Could you check a few things on this drawing? It's one solid part, dimensions in mm from its lowest x, y, z. A direction names the side the tool comes from. Give positions to 0.01 mm unless a question says otherwise; leave off trailing zeros. Loops run counter-clockwise (first coordinate to the right, second up) from the corner with the lowest first, then second, coordinate; pieces in that order, holes last.
Q1. Suppose I cut it at C-C (y = 1.6). List the corners of the cut face in (x, z) for me.
Q2. Suppose I cut it at D-D (x = 18.5). List the corners of the cut face in (y, z) for me.
Q3. Suppose I cut it at B-B (x = 3.5). List the corners of the cut face in (y, z) for me, and give its area (3 significant figures).
Q4. I need wall thicknesses on probe 1 along X at (y, z) = (1.6, 3.5); probe 2 along Z at (x, y) = (22, 1.8); probe 3 along X at (y, z) = (0.9, 6.5). Which ranges of each line are inside material? Lowest first, please.
Q5. Thinking about a two-plate mould opening in X: for the marked faces 1 and 2, which applies, pulls with the +X half, pulls with the -X half, needs draft (parallel to the pull), parting line crosses it, or undercut?
Q6. Suppose I cut it at A-A (z = 3.5). List the corners of the cut face in (x, y) for me, and give its area (3 significant figures).
Q7. I'm going to push flat-ended pins straight in: P1, Ø2, axis at x = 8.5, z = 4, coming from the -Y side; P2, Ø5, axis at x = 26, z = 9, coming from the +Y side. Where does each tip first touch, or does it pass through?
Q8. For the marked faces 3 and 4, which set-ups out of +Z, -Z, +X, -X, +Y, -Y let a thin tool reach every point of the face, with its end or its side?
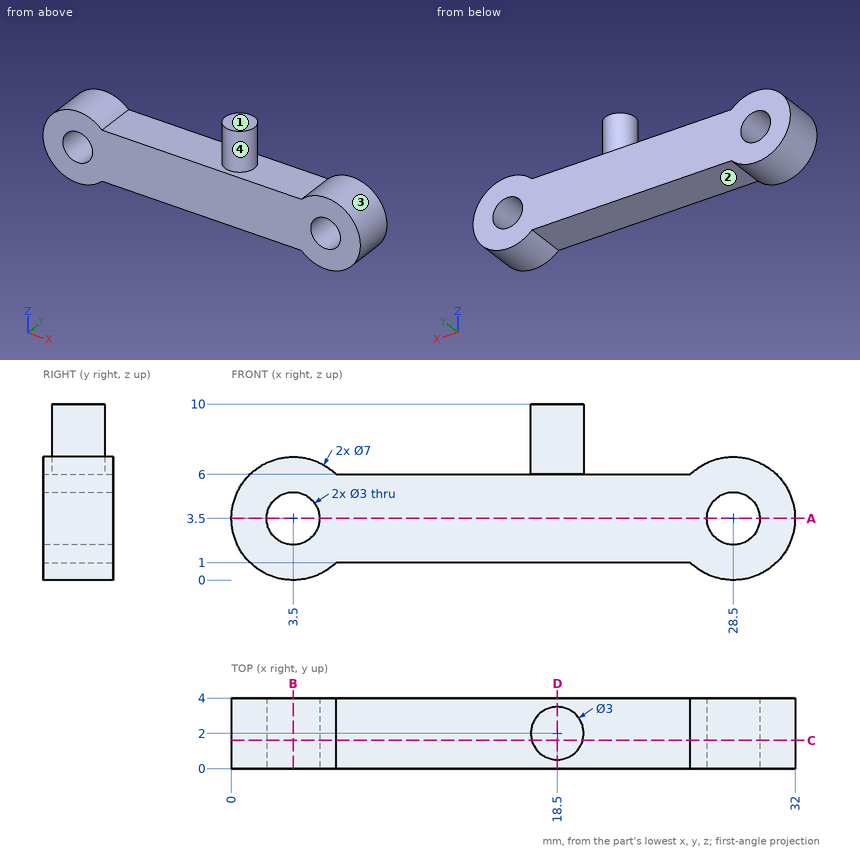
Solutions:
1. outline: (5.95, 1) - (26.05, 1) arc R3.5 ccw (long way) to (26.05, 6) - (19.95, 6) - (19.95, 10) - (17.05, 10) - (17.05, 6) - (5.95, 6) arc R3.5 ccw (long way) to start; hole circle Ø3 at (3.5, 3.5); hole circle Ø3 at (28.5, 3.5)
2. outline: (0, 1) - (4, 1) - (4, 6) - (3.5, 6) - (3.5, 10) - (0.5, 10) - (0.5, 6) - (0, 6) - close
3. outline: (0, 0) - (4, 0) - (4, 2) - (0, 2) - close; (0, 5) - (4, 5) - (4, 7) - (0, 7) - close
3. area: 16.0 mm2
4. probe 1: x = 0 to 2, 5 to 27, 30 to 32
4. probe 2: z = 1 to 6
4. probe 3: x = 1.7 to 5.3, 17.48 to 19.52, 26.7 to 30.3
5. face 1: needs draft
5. face 2: undercut
6. outline: (0, 0) - (2, 0) - (2, 4) - (0, 4) - close; (5, 0) - (27, 0) - (27, 4) - (5, 4) - close; (30, 0) - (32, 0) - (32, 4) - (30, 4) - close
6. area: 104 mm2
7. P1: stops at y = 0
7. P2: passes through
8. face 3: +Y, -Y
8. face 4: +Z
